Model file for the job. Use its own axes, mm. A direction names the side the tool comes from. Round coordinates to 2 decimals unless told otherwise and drop trailing zeros. Order: outer loops, then holes, each group sorted by start corner. A loop starts at its lowest first (then second) coordinate and runs counter-clockwise, first axis right, second up. Notation, with made-up numbers: (-34, -3.75) - (-18, -3.75) arc R3 cw to (-18, 0.25) - close; hole circle Ø2 at (35, 58). An arc over 180 degrees is marked (long way). Put each result on its own line as item: value. Start each with the question number.
Item 1: Mould opens along Y. For faces 4 (the face through (-4, 77.938, -2)), 5 (the face through (-3.913, 43.091, -46.762)), 6 (the face through (126.695, 3.913, -92.298)) say: pulls with the +Y half, pulls with the -Y half, needs draft (parallel to the pull), parting line crosses it, or undercut.
Item 2: Probe probe 1 along X at (y, z) = (71, -1); probe 2 along Y at (x, z) = (58, -86.5); probe 3 along X at (y, z) = (11.5, 80.5). List the from-to ranges inside material, lowest first.
Item 3: Which spindle directions (+Z, -Z, +X, -X, +Y, -Y) get a long thin tool onto all of the face, cutting with end or side? Do faces 1 (the face through (-4, 49.938, 89)), 2 (the face through (41.5, 4, 90)), 3 (the face through (14, 7, 145)). Say none if no direction does.
Item 4: Saw through at C-C on x = 104. List the corners of the cut face in (y, z), plus the area to 3 significant figures.
Item 5: Saw through at D-D on z = 19. List the corners of the cut face in (x, y) (1 decimal).
Item 6: Saw through at A-A on x = 35. List the corners of the cut face in (y, z).
Item 7: Pin check, flat tips, straight feed: pin 1 Ø10 at (y, z) = (49, -31) entering from +X; pin 2 Ø8.5 at (x, y) = (140.5, 5.5) entering from +Z; pin 3 Ø2.5 at (x, z) = (-4, -103.5) entering from -Y. Stop position of each tip, or through.
Item 8: Saw through at B-B on z = 111.5. List the corners of the cut face in (x, y) (1 decimal), plus the area to 3 significant figures.
```python
from build123d import *

# Parameters (mm, degrees)
SALIENTE_EXTRUIR1_DEPTH   = 7.9375
CROQUIS2_W                = 290
CROQUIS2_H                = 77.9375
SALIENTE_EXTRUIR2_DEPTH   = 7.9375
CONVERTIR_S_LIDO1_START   = -145
CONVERTIR_S_LIDO1_DEPTH   = 290
CONVERTIR_S_LIDO1_2_DEPTH = 290


# Read off the part's stored shape, not the designer's step: Convertir-Sólido1
with BuildPart() as part:
    # Croquis1 → Saliente-Extruir1 (new body)
    with BuildSketch(Plane(origin=(0, 0, 0), x_dir=(1, 0, 0), z_dir=(0, 1, 0))):
        Polygon((70, -145), (0, -145), (0, 145), (70, 145), (185, 38.1), (185, -38.1), align=None)
        with BuildLine():
            ThreePointArc((41.5, -80), (35, -73.5), (28.5, -80))
            Line((28.5, -80), (28.5, -100))
            ThreePointArc((28.5, -100), (35, -106.5), (41.5, -100))
            Line((41.5, -100), (41.5, -80))
        make_face(mode=Mode.SUBTRACT)
        with BuildLine():
            ThreePointArc((160, -7.597922996), (167.597922996, 0), (160, 7.597922996))
            Line((160, 7.597922996), (100, 7.597922996))
            ThreePointArc((100, 7.597922996), (92.402077004, 0), (100, -7.597922996))
            Line((100, -7.597922996), (160, -7.597922996))
        make_face(mode=Mode.SUBTRACT)
        with BuildLine():
            Line((41.5, 100), (41.5, 80))
            ThreePointArc((41.5, 80), (35, 73.5), (28.5, 80))
            Line((28.5, 80), (28.5, 100))
            ThreePointArc((28.5, 100), (35, 106.5), (41.5, 100))
        make_face(mode=Mode.SUBTRACT)
    extrude(amount=SALIENTE_EXTRUIR1_DEPTH)

    # Croquis2 → Saliente-Extruir2 (add)
    with BuildSketch(Plane.ZY):
        with Locations((0, 38.96875)):
            Rectangle(CROQUIS2_W, CROQUIS2_H)
        with BuildLine():
            ThreePointArc((-125, 35.9375), (-132, 42.9375), (-125, 49.9375))
            Line((-125, 49.9375), (-53.76065494, 49.9375))
            ThreePointArc((-53.76065494, 49.9375), (-46.76065494, 42.9375), (-53.76065494, 35.9375))
            Line((-53.76065494, 35.9375), (-125, 35.9375))
        make_face(mode=Mode.SUBTRACT)
        with BuildLine():
            Line((53.76065494, 49.9375), (125, 49.9375))
            ThreePointArc((125, 49.9375), (132, 42.9375), (125, 35.9375))
            Line((125, 35.9375), (53.76065494, 35.9375))
            ThreePointArc((53.76065494, 35.9375), (46.76065494, 42.9375), (53.76065494, 49.9375))
        make_face(mode=Mode.SUBTRACT)
    extrude(amount=SALIENTE_EXTRUIR2_DEPTH)

    # Convertir-Sólido1 outline → Convertir-Sólido1 (cut)
    with BuildSketch(Plane.XY.offset(CONVERTIR_S_LIDO1_START)):
        with BuildLine():
            Line((-7.9375, 0), (8, 0))
            ThreePointArc((8, 0), (-3.269514325, 4.667985675), (-7.9375, 15.9375))
            Line((-7.9375, 15.9375), (-7.9375, 0))
        make_face()
    extrude(amount=CONVERTIR_S_LIDO1_DEPTH, mode=Mode.SUBTRACT)

    # Convertir-S_lido1 2 outline → Convertir-S_lido1 2 (add)
    with BuildSketch(Plane.XY.offset(CONVERTIR_S_LIDO1_START)):
        with BuildLine():
            Line((0, 7.9375), (8, 7.9375))
            ThreePointArc((8, 7.9375), (2.343145751, 10.280645751), (0, 15.9375))
            Line((0, 15.9375), (0, 7.9375))
        make_face()
    extrude(amount=CONVERTIR_S_LIDO1_2_DEPTH)


solid = part.part
```
Results found:
1. face 4: pulls with the +Y half
1. face 5: undercut
1. face 6: needs draft
2. probe 1: x = -7.94 to 0
2. probe 2: y = 0 to 7.94
2. probe 3: x = -7.31 to 1.34
3. face 1: +X, -X
3. face 2: +Y, -Y
3. face 3: +Z, +X, -X, +Y, -Y
4. outline: (0, -113.39) - (7.94, -113.39) - (7.94, -7.6) - (0, -7.6) - close; (0, 7.6) - (7.94, 7.6) - (7.94, 113.39) - (0, 113.39) - close
4. area: 1,680 mm²
5. outline: (-7.9, 15.9) arc R15.9 ccw to (8, 0) - (185, 0) - (185, 7.9) - (8, 7.9) arc R8 cw to (0, 15.9) - (0, 77.9) - (-7.9, 77.9) - close
6. outline: (0, -145) - (7.94, -145) - (7.94, -106.5) - (0, -106.5) - close; (0, -73.5) - (7.94, -73.5) - (7.94, 73.5) - (0, 73.5) - close; (0, 106.5) - (7.94, 106.5) - (7.94, 145) - (0, 145) - close
7. pin 1: stops at x = 0
7. pin 2: stops at z = 83.42
7. pin 3: stops at y = 4.17
8. outline: (-7.9, 15.9) arc R15.9 ccw to (8, 0) - (106, 0) - (106, 7.9) - (8, 7.9) arc R8 cw to (0, 15.9) - (0, 35.9) - (-7.9, 35.9) - close; (-7.9, 49.9) - (0, 49.9) - (0, 77.9) - (-7.9, 77.9) - close
8. area: 1,310 mm²
